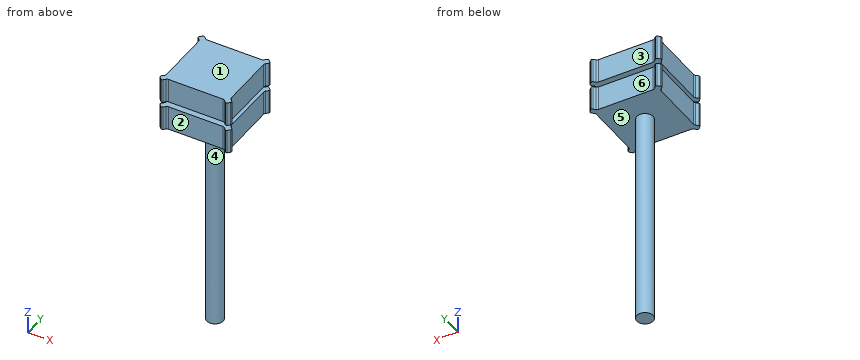
from build123d import *

# Parameters (mm, degrees)
BOSS_EXTRUDE1_DEPTH = 20
SKETCH3_R           = 3
BOSS_EXTRUDE2_DEPTH = 80
SKETCH5_R           = 20
SKETCH5_R_2         = 4
CUT_EXTRUDE1_DEPTH  = 2


with BuildPart() as part:
    # Sketch1 → Boss-Extrude1 (new body)
    with BuildSketch(Plane.XY):
        with BuildLine():
            Line((-13.060660172, 11.560660172), (-12.292893219, 10.792893219))
            ThreePointArc((-12.292893219, 10.792893219), (-12.076120467, 10.46846987), (-12, 10.085786438))
            Line((-12, 10.085786438), (-12, -10.085786438))
            ThreePointArc((-12, -10.085786438), (-12.076120467, -10.46846987), (-12.292893219, -10.792893219))
            Line((-12.292893219, -10.792893219), (-13.060660172, -11.560660172))
            ThreePointArc((-13.060660172, -11.560660172), (-13.207106781, -11.914213562), (-13.060660172, -12.267766953))
            Line((-13.060660172, -12.267766953), (-12.267766953, -13.060660172))
            ThreePointArc((-12.267766953, -13.060660172), (-11.914213562, -13.207106781), (-11.560660172, -13.060660172))
            Line((-11.560660172, -13.060660172), (-10.792893219, -12.292893219))
            ThreePointArc((-10.792893219, -12.292893219), (-10.46846987, -12.076120467), (-10.085786438, -12))
            Line((-10.085786438, -12), (10.085786438, -12))
            ThreePointArc((10.085786438, -12), (10.46846987, -12.076120467), (10.792893219, -12.292893219))
            Line((10.792893219, -12.292893219), (11.560660172, -13.060660172))
            ThreePointArc((11.560660172, -13.060660172), (11.914213562, -13.207106781), (12.267766953, -13.060660172))
            Line((12.267766953, -13.060660172), (13.060660172, -12.267766953))
            ThreePointArc((13.060660172, -12.267766953), (13.207106781, -11.914213562), (13.060660172, -11.560660172))
            Line((13.060660172, -11.560660172), (12.292893219, -10.792893219))
            ThreePointArc((12.292893219, -10.792893219), (12.076120467, -10.46846987), (12, -10.085786438))
            Line((12, -10.085786438), (12, 10.085786438))
            ThreePointArc((12, 10.085786438), (12.076120467, 10.46846987), (12.292893219, 10.792893219))
            Line((12.292893219, 10.792893219), (13.060660172, 11.560660172))
            ThreePointArc((13.060660172, 11.560660172), (13.207106781, 11.914213562), (13.060660172, 12.267766953))
            Line((13.060660172, 12.267766953), (12.267766953, 13.060660172))
            ThreePointArc((12.267766953, 13.060660172), (11.914213562, 13.207106781), (11.560660172, 13.060660172))
            Line((11.560660172, 13.060660172), (10.792893219, 12.292893219))
            ThreePointArc((10.792893219, 12.292893219), (10.46846987, 12.076120467), (10.085786438, 12))
            Line((10.085786438, 12), (-10.085786438, 12))
            ThreePointArc((-10.085786438, 12), (-10.46846987, 12.076120467), (-10.792893219, 12.292893219))
            Line((-10.792893219, 12.292893219), (-11.560660172, 13.060660172))
            ThreePointArc((-11.560660172, 13.060660172), (-11.914213562, 13.207106781), (-12.267766953, 13.060660172))
            Line((-12.267766953, 13.060660172), (-13.060660172, 12.267766953))
            ThreePointArc((-13.060660172, 12.267766953), (-13.207106781, 11.914213562), (-13.060660172, 11.560660172))
        make_face()
    extrude(amount=BOSS_EXTRUDE1_DEPTH)

    # Sketch3 → Boss-Extrude2 (add)
    with BuildSketch(Plane(origin=(0, 0, 0), x_dir=(-1, 0, 0), z_dir=(0, 0, -1))):
        Circle(SKETCH3_R)
    extrude(amount=BOSS_EXTRUDE2_DEPTH)

    # Sketch5 → Cut-Extrude1 (cut)
    with BuildSketch(Plane.XY.offset(11)):
        Circle(SKETCH5_R)
        Circle(SKETCH5_R_2, mode=Mode.SUBTRACT)
    extrude(amount=-CUT_EXTRUDE1_DEPTH, mode=Mode.SUBTRACT)


solid = part.part
Verification items for the finished model (mm, model axes). Face numbers are marked on the shaded views. A direction names the side the tool comes from. Coordinates: 2 decimals unless noted, no trailing zeros. Order: outer loops, then holes, each group sorted by start corner. A loop starts at its lowest first (then second) coordinate and runs counter-clockwise, first axis right, second up. Notation, with made-up numbers: (4, 74) -> (58, 74) arc R16 cw to (58, 81) -> close; hole circle Ø6 at (51, 89.25). An arc over 180 degrees is marked (long way). Put each result on its own line as item: value. Start each with the question number.
1. Go/stop test with flat-tipped pins: pin 1 Ø4.5 at (x, z) = (0, 15) entering from -Y; pin 2 Ø1 at (y, z) = (8, 2.5) entering from +X; pin 3 Ø4 at (x, y) = (10, -6.5) entering from -Z. Record where each tip stops, or that it passes through.
2. Cross-section at D-D, the plane z = -17.5. Record the boundary of the cut face in (x, y).
3. Cross-section at A-A, the plane x = -9. Record the boundary of the cut face in (y, z).
4. Material ranges on L1, parallel to Z at x = -7.75, y = -5; L2, parallel to Y at x = 0.25, z = 10; L3, parallel to Y at x = -8, z = 2, recorded low to high. Write a range as [from, to].
5. Cross-section at B-B, the plane y = 0. Record the boundary of the cut face in (x, z), then the cut area to 3 significant figures.
6. Mould release check, pull along X, two halves, no side actions. Record for the marked faces 4, 5 and 6: released by +X, released by -X, zero draft, split by the parting line, or undercut.
7. Access from +Z, -Z, +X, -X, +Y, -Y to the whole of each face (thin tool, end or side, straight path). Record for the marked faces 1, 2 and 3.
Computed:
1. pin 1: y = -12
1. pin 2: x = 12
1. pin 3: z = 0
2. outline: circle Ø6 at (0, 0)
3. outline: (-12, 0) -> (12, 0) -> (12, 9) -> (-12, 9) -> close; (-12, 11) -> (12, 11) -> (12, 20) -> (-12, 20) -> close
4. L1: [0, 9], [11, 20]
4. L2: [-3.99, 3.99]
4. L3: [-12, 12]
5. outline: (-12, 0) -> (-3, 0) -> (-3, -80) -> (3, -80) -> (3, 0) -> (12, 0) -> (12, 9) -> (4, 9) -> (4, 11) -> (12, 11) -> (12, 20) -> (-12, 20) -> (-12, 11) -> (-4, 11) -> (-4, 9) -> (-12, 9) -> close
5. area: 928 mm2
6. face 4: split by the parting line
6. face 5: zero draft
6. face 6: undercut
7. face 1: +Z, +X, -X, +Y, -Y
7. face 2: +Z, -Z, -Y
7. face 3: +Z, -Z, +Y
